Source: CAD feature listing. Evaluate the final solid. Frame: model axes, mm. Face numbers are marked on the shaded views. Coordinates: 2 decimals unless noted, no trailing zeros. Loops run counter-clockwise (first coordinate to the right, second up) from the corner with the lowest first, then second, coordinate; pieces in that order, holes last. Notation, with made-up numbers: (25, 87) - (75, 87) arc R23 ccw to (75, 126) - close; hole circle Ø8 at (54, 61.25). An arc over 180 degrees is marked (long way). Use one line per item in the form item = value. Start each with the question number.
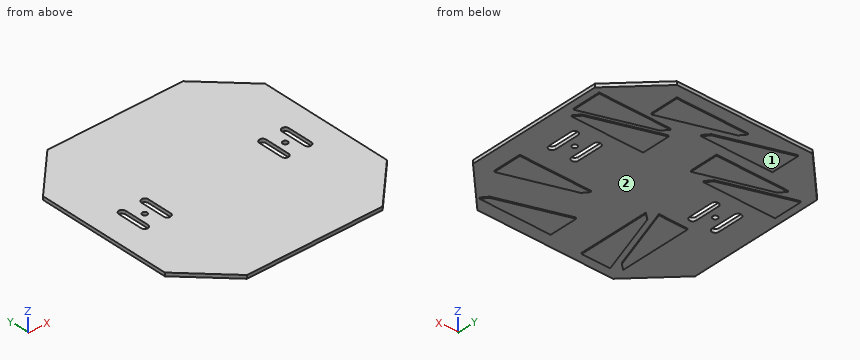
from build123d import *

# Parameters (mm, degrees)
BOSS_EXTRUDE1_OUTLINE_R  = 1.1
BOSS_EXTRUDE1_DEPTH      = 1.5
BOSS_EXTRUDE2_DEPTH      = 1.5
BOSS_EXTRUDE2_DEPTH_BACK = 0.5


# Read off the part's stored shape, not the designer's step: Boss-Extrude1
with BuildPart() as part:
    # Boss-Extrude1 outline → Boss-Extrude1 (new body)
    with BuildSketch(Plane.XY):
        Polygon((19.1, 98), (0, 78.9), (0, 19.1), (19.1, 0), (78.9, 0), (98, 19.1), (98, 78.9), (78.9, 98), align=None)
        with BuildLine():
            Line((36.8757, 35.879), (36.857308756, 4.446264405))
            ThreePointArc((36.857308756, 4.446264405), (36.875994273, 4.43215571), (36.879898885, 4.409069831))
            ThreePointArc((36.879898885, 4.409069831), (36.853148575, 4.399873011), (36.829703907, 4.41570046))
            Line((36.829703907, 4.41570046), (24.3261, 4.416))
            Line((24.3261, 4.416), (34.2414, 33.6881))
            Line((34.2414, 33.6881), (36.8757, 35.879))
        make_face(mode=Mode.SUBTRACT)
        with BuildLine():
            Line((20.5443, 6.661), (20.562691244, 38.093735595))
            ThreePointArc((20.562691244, 38.093735595), (20.544005727, 38.10784429), (20.540101115, 38.130930169))
            ThreePointArc((20.540101115, 38.130930169), (20.566851425, 38.140126989), (20.590296093, 38.12429954))
            Line((20.590296093, 38.12429954), (33.0939, 38.124))
            Line((33.0939, 38.124), (23.1786, 8.8519))
            Line((23.1786, 8.8519), (20.5443, 6.661))
        make_face(mode=Mode.SUBTRACT)
        with BuildLine():
            Line((11.5, 43.5), (11.5, 54.5))
            ThreePointArc((11.5, 54.5), (13, 56), (14.5, 54.5))
            Line((14.5, 54.5), (14.5, 43.5))
            ThreePointArc((14.5, 43.5), (13, 42), (11.5, 43.5))
        make_face(mode=Mode.SUBTRACT)
        with Locations((18, 49)):
            Circle(BOSS_EXTRUDE1_OUTLINE_R, mode=Mode.SUBTRACT)
        with BuildLine():
            Line((21.5, 43.5), (21.5, 54.5))
            ThreePointArc((21.5, 54.5), (23, 56), (24.5, 54.5))
            Line((24.5, 54.5), (24.5, 43.5))
            ThreePointArc((24.5, 43.5), (23, 42), (21.5, 43.5))
        make_face(mode=Mode.SUBTRACT)
        with BuildLine():
            Line((83.379, 5.9243), (51.946264405, 5.942691244))
            ThreePointArc((51.946264405, 5.942691244), (51.93215571, 5.924005727), (51.909069831, 5.920101115))
            ThreePointArc((51.909069831, 5.920101115), (51.899873011, 5.946851425), (51.91570046, 5.970296093))
            Line((51.91570046, 5.970296093), (51.916, 18.4739))
            Line((51.916, 18.4739), (81.1881, 8.5586))
            Line((81.1881, 8.5586), (83.379, 5.9243))
        make_face(mode=Mode.SUBTRACT)
        with BuildLine():
            Line((58.661, 33.3357), (90.093735595, 33.317308756))
            ThreePointArc((90.093735595, 33.317308756), (90.10784429, 33.335994273), (90.130930169, 33.339898885))
            ThreePointArc((90.130930169, 33.339898885), (90.140126989, 33.313148575), (90.12429954, 33.289703907))
            Line((90.12429954, 33.289703907), (90.124, 20.7861))
            Line((90.124, 20.7861), (60.8519, 30.7014))
            Line((60.8519, 30.7014), (58.661, 33.3357))
        make_face(mode=Mode.SUBTRACT)
        with BuildLine():
            Line((73.5, 43.5), (73.5, 54.5))
            ThreePointArc((73.5, 54.5), (75, 56), (76.5, 54.5))
            Line((76.5, 54.5), (76.5, 43.5))
            ThreePointArc((76.5, 43.5), (75, 42), (73.5, 43.5))
        make_face(mode=Mode.SUBTRACT)
        with Locations((80, 49)):
            Circle(BOSS_EXTRUDE1_OUTLINE_R, mode=Mode.SUBTRACT)
        with BuildLine():
            Line((83.5, 43.5), (83.5, 54.5))
            ThreePointArc((83.5, 54.5), (85, 56), (86.5, 54.5))
            Line((86.5, 54.5), (86.5, 43.5))
            ThreePointArc((86.5, 43.5), (85, 42), (83.5, 43.5))
        make_face(mode=Mode.SUBTRACT)
        with BuildLine():
            Line((35.009, 62.2543), (3.576264405, 62.272691244))
            ThreePointArc((3.576264405, 62.272691244), (3.56215571, 62.254005727), (3.539069831, 62.250101115))
            ThreePointArc((3.539069831, 62.250101115), (3.529873011, 62.276851425), (3.54570046, 62.300296093))
            Line((3.54570046, 62.300296093), (3.546, 74.8039))
            Line((3.546, 74.8039), (32.8181, 64.8886))
            Line((32.8181, 64.8886), (35.009, 62.2543))
        make_face(mode=Mode.SUBTRACT)
        with BuildLine():
            Line((10.751, 76.5657), (42.183735595, 76.547308756))
            ThreePointArc((42.183735595, 76.547308756), (42.19784429, 76.565994273), (42.220930169, 76.569898885))
            ThreePointArc((42.220930169, 76.569898885), (42.230126989, 76.543148575), (42.21429954, 76.519703907))
            Line((42.21429954, 76.519703907), (42.214, 64.0161))
            Line((42.214, 64.0161), (12.9419, 73.9314))
            Line((12.9419, 73.9314), (10.751, 76.5657))
        make_face(mode=Mode.SUBTRACT)
        with BuildLine():
            Line((53.599, 81.6043), (22.166264405, 81.622691244))
            ThreePointArc((22.166264405, 81.622691244), (22.15215571, 81.604005727), (22.129069831, 81.600101115))
            ThreePointArc((22.129069831, 81.600101115), (22.119873011, 81.626851425), (22.13570046, 81.650296093))
            Line((22.13570046, 81.650296093), (22.136, 94.1539))
            Line((22.136, 94.1539), (51.4081, 84.2386))
            Line((51.4081, 84.2386), (53.599, 81.6043))
        make_face(mode=Mode.SUBTRACT)
        with BuildLine():
            Line((92.809, 61.7843), (61.376264405, 61.802691244))
            ThreePointArc((61.376264405, 61.802691244), (61.36215571, 61.784005727), (61.339069831, 61.780101115))
            ThreePointArc((61.339069831, 61.780101115), (61.329873011, 61.806851425), (61.34570046, 61.830296093))
            Line((61.34570046, 61.830296093), (61.346, 74.3339))
            Line((61.346, 74.3339), (90.6181, 64.4186))
            Line((90.6181, 64.4186), (92.809, 61.7843))
        make_face(mode=Mode.SUBTRACT)
        with BuildLine():
            Line((63.531, 77.7357), (94.963735595, 77.717308756))
            ThreePointArc((94.963735595, 77.717308756), (94.97784429, 77.735994273), (95.000930169, 77.739898885))
            ThreePointArc((95.000930169, 77.739898885), (95.010126989, 77.713148575), (94.99429954, 77.689703907))
            Line((94.99429954, 77.689703907), (94.994, 65.1861))
            Line((94.994, 65.1861), (65.7219, 75.1014))
            Line((65.7219, 75.1014), (63.531, 77.7357))
        make_face(mode=Mode.SUBTRACT)
        with BuildLine():
            Line((42.721, 92.6557), (74.153735595, 92.637308756))
            ThreePointArc((74.153735595, 92.637308756), (74.16784429, 92.655994273), (74.190930169, 92.659898885))
            ThreePointArc((74.190930169, 92.659898885), (74.200126989, 92.633148575), (74.18429954, 92.609703907))
            Line((74.18429954, 92.609703907), (74.184, 80.1061))
            Line((74.184, 80.1061), (44.9119, 90.0214))
            Line((44.9119, 90.0214), (42.721, 92.6557))
        make_face(mode=Mode.SUBTRACT)
    extrude(amount=BOSS_EXTRUDE1_DEPTH)

    # Model<4> → Boss-Extrude2 (add, two sides: drawn at the far end of the back side and taken through both)
    with BuildSketch(Plane.XY.offset(-BOSS_EXTRUDE2_DEPTH_BACK)):
        Polygon((42.2143, 76.5473), (42.1987, 76.5473), (42.183735595, 76.547308756), (10.751, 76.5657), (12.92157794, 73.955834891), (12.9419, 73.9314), (12.971962529, 73.921216959), (42.214, 64.0161), (42.21429954, 76.519703907), (42.2143, 76.5389), align=None)
        Polygon((3.54570046, 62.300296093), (3.5457, 62.2811), (3.5457, 62.2727), (3.5613, 62.2727), (3.576264405, 62.272691244), (35.009, 62.2543), (32.83842206, 64.864165109), (32.8181, 64.8886), (32.788037471, 64.898783041), (3.546, 74.8039), align=None)
        Polygon((22.13570046, 81.650296093), (22.1357, 81.6311), (22.1357, 81.623120089), (22.1513, 81.6227), (22.166264405, 81.622691244), (53.599, 81.6043), (51.42842206, 84.214165109), (51.4081, 84.2386), (51.378037471, 84.248783041), (22.136, 94.1539), align=None)
        Polygon((74.1843, 92.6373), (74.1687, 92.6373), (74.153735595, 92.637308756), (42.721, 92.6557), (44.89157794, 90.045834891), (44.9119, 90.0214), (44.941962529, 90.011216959), (74.184, 80.1061), (74.18429954, 92.609703907), (74.1843, 92.6289), align=None)
        Polygon((94.9943, 77.7173), (94.9787, 77.7173), (94.963735595, 77.717308756), (63.531, 77.7357), (65.70157794, 75.125834891), (65.7219, 75.1014), (65.751962529, 75.091216959), (94.994, 65.1861), (94.99429954, 77.689703907), (94.9943, 77.7089), align=None)
        Polygon((61.34570046, 61.830296093), (61.3457, 61.8111), (61.3457, 61.8027), (61.3613, 61.8027), (61.376264405, 61.802691244), (92.809, 61.7843), (90.63842206, 64.394165109), (90.6181, 64.4186), (90.588037471, 64.428783041), (61.346, 74.3339), align=None)
        Polygon((20.5627, 38.1243), (20.5627, 38.1087), (20.562691244, 38.093735595), (20.5443, 6.661), (23.154165109, 8.83157794), (23.1786, 8.8519), (23.188783041, 8.881962529), (33.0939, 38.124), (20.590296093, 38.12429954), (20.5711, 38.1243), align=None)
        Polygon((36.8573, 4.4157), (36.8573, 4.4313), (36.857308756, 4.446264405), (36.8757, 35.879), (34.265834891, 33.70842206), (34.2414, 33.6881), (34.231216959, 33.658037471), (24.3261, 4.416), (36.829703907, 4.41570046), (36.8489, 4.4157), align=None)
        Polygon((51.91570046, 5.970296093), (51.9157, 5.9511), (51.9157, 5.9427), (51.9313, 5.9427), (51.946264405, 5.942691244), (83.379, 5.9243), (81.20842206, 8.534165109), (81.1881, 8.5586), (81.158037471, 8.568783041), (51.916, 18.4739), align=None)
        Polygon((90.1243, 33.3173), (90.1087, 33.3173), (90.093735595, 33.317308756), (58.661, 33.3357), (60.83157794, 30.725834891), (60.8519, 30.7014), (60.881962529, 30.691216959), (90.124, 20.7861), (90.12429954, 33.289703907), (90.1243, 33.3089), align=None)
    extrude(amount=BOSS_EXTRUDE2_DEPTH + BOSS_EXTRUDE2_DEPTH_BACK)


solid = part.part
(1) Cut plane A-A, the plane y = 53. Output: boundary loops of the cut face in (x, z).
(2) Contact query for a flat-ended pin moving along its axis: pin 1 (2 mm diameter, centred on x = 47.5, y = 30, fed in from -Z). Output: stop coordinate, or through.
(3) Material intervals for line 1 (X direction, y = 47, z = 0.7); line 2 (Y direction, x = 52, z = -0.05); line 3 (Y direction, x = 18, z = 0.8), sorted ascending.
(4) Mould query, pull axis Y, two halves, no side actions, for the marked faces 1 and 2. Classes: +Y half, -Y half, draft (parallel to the pull), parting line (faces both ways), or undercut.
(5) Cut plane B-B, the plane x = 85. Output: boundary loops of the cut face in (y, z).
(6) Cut plane D-D, the plane x = 40.5. Output: boundary loops of the cut face in (y, z).
Recorded:
q1.outline = (0, 0) - (11.5, 0) - (11.5, 1.5) - (0, 1.5) - close; (14.5, 0) - (21.5, 0) - (21.5, 1.5) - (14.5, 1.5) - close; (24.5, 0) - (73.5, 0) - (73.5, 1.5) - (24.5, 1.5) - close; (76.5, 0) - (83.5, 0) - (83.5, 1.5) - (76.5, 1.5) - close; (86.5, 0) - (98, 0) - (98, 1.5) - (86.5, 1.5) - close
q2.pin_1 = 0
q3.line_1 = 0 to 11.5, 14.5 to 21.5, 24.5 to 73.5, 76.5 to 83.5, 86.5 to 98
q3.line_2 = 5.94 to 18.45, 81.61 to 83.53, 87.62 to 92.65
q3.line_3 = 1.1 to 47.9, 50.1 to 96.9
q4.face_1 = draft
q4.face_2 = undercut
q5.outline = (6.1, 0) - (22.52, 0) - (22.52, -0.5) - (33.32, -0.5) - (33.32, 0) - (42, 0) - (42, 1.5) - (6.1, 1.5) - close; (56, 0) - (61.79, 0) - (61.79, -0.5) - (66.32, -0.5) - (66.32, 0) - (68.57, 0) - (68.57, -0.5) - (77.72, -0.5) - (77.72, 0) - (91.9, 0) - (91.9, 1.5) - (56, 1.5) - close
q6.outline = (0, 0) - (64.6, 0) - (64.6, -0.5) - (76.55, -0.5) - (76.55, 0) - (81.61, 0) - (81.61, -0.5) - (87.93, -0.5) - (87.93, 0) - (98, 0) - (98, 1.5) - (0, 1.5) - close
